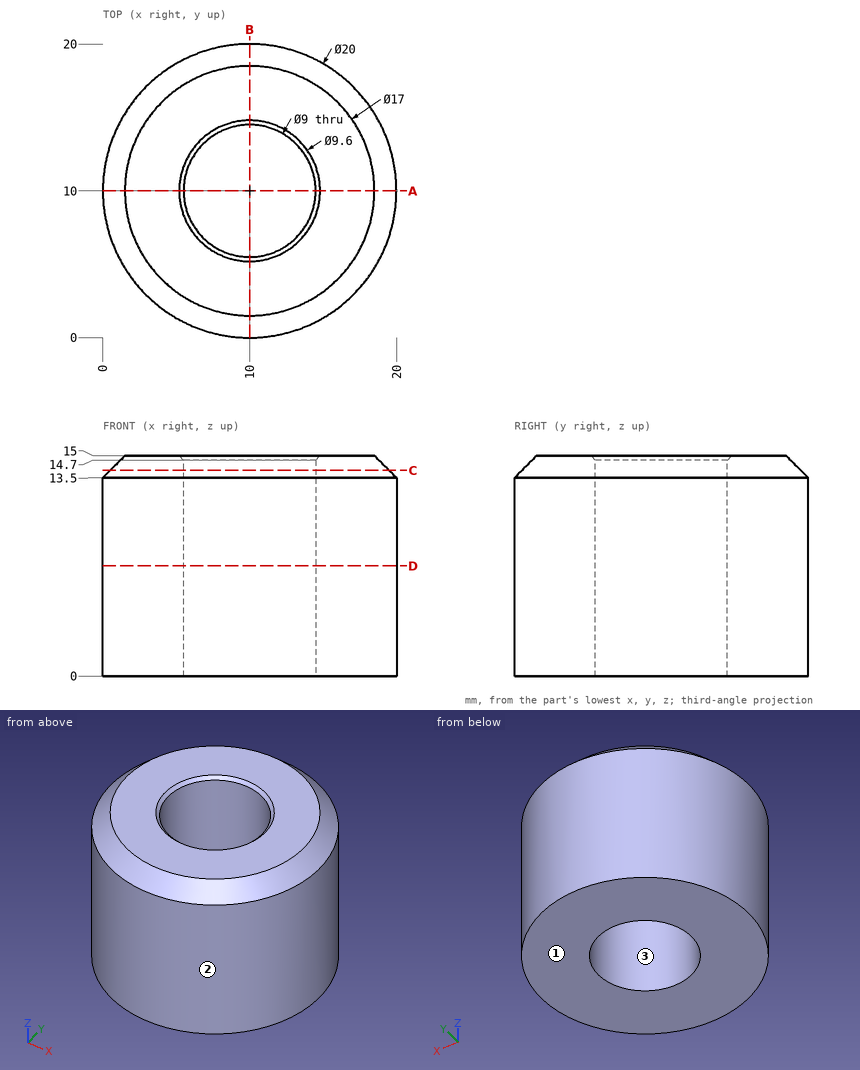
Drawing for the job (mm, zero at the part's lowest x, y, z). Coordinates: 2 decimals unless noted, no trailing zeros. Write each loop counter-clockwise with the first axis right and the second up, starting at its lowest first coordinate (ties: lowest second). Pieces come first, ordered by that corner, then holes. Notation, with made-up numbers: (67.5, 71.5) -> (117.5, 71.5) arc R6 ccw to (117.5, 82.5) -> close; hole circle Ø10 at (-11, 36.5). An arc over 180 degrees is marked (long way). One line per item, written item: value. Start each with the question number.
1) Slice it at C-C on z = 14. Write the cut outline in (x, y), then the cut area to 3 significant figures.
2) Flat gauge pins, fed straight in: pin 1 Ø3 at (x, z) = (7.5, 9.5) entering from +Y; pin 2 Ø4 at (y, z) = (3, 10.5) entering from -X. Where does each tip first touch, or does it go through?
3) Slice it at D-D on z = 7.5. Write the cut outline in (x, y).
4) Probe probe 1 along Y at (x, z) = (10, 5.75); probe 2 along Y at (x, z) = (13, 12.75); probe 3 along X at (y, z) = (9, 0.75). List the from-to ranges inside material, lowest first.
5) Pull direction Y, two halves, no side cores. Call the marked faces 1, 2 and 3: +Y half, -Y half, draft (parallel to the pull), parting line (faces both ways), or undercut.
6) Slice it at A-A on y = 10. Write the cut outline in (x, z), then the cut area to 3 significant figures.
Answers follow:
1. outline: circle Ø19 at (10, 10); hole circle Ø9 at (10, 10)
1. area: 220 mm2
2. pin 1: y = 19.95
2. pin 2: x = 1.34
3. outline: circle Ø20 at (10, 10); hole circle Ø9 at (10, 10)
4. probe 1: 0 to 5.5, 14.5 to 20
4. probe 2: 0.46 to 6.65, 13.35 to 19.54
4. probe 3: 0.05 to 5.61, 14.39 to 19.95
5. face 1: draft
5. face 2: parting line
5. face 3: undercut
6. outline: (0, 0) -> (5.5, 0) -> (5.5, 14.7) -> (5.2, 15) -> (1.5, 15) -> (0, 13.5) -> close; (14.5, 0) -> (20, 0) -> (20, 13.5) -> (18.5, 15) -> (14.8, 15) -> (14.5, 14.7) -> close
6. area: 163 mm2
